For this review, use the dimensioned drawing (mm, ordinates from the lowest corner) and the shaded views. Coordinates: 2 decimals unless noted, no trailing zeros. Loops run counter-clockwise (first coordinate to the right, second up) from the corner with the lowest first, then second, coordinate; pieces in that order, holes last. Notation, with made-up numbers: M 14,62.25 L 32,62.25 A18 ccw 32,87.25 Z; hole C 30.25,79 d2. An arc over 180 degrees is marked long. Write item = value, one per line.
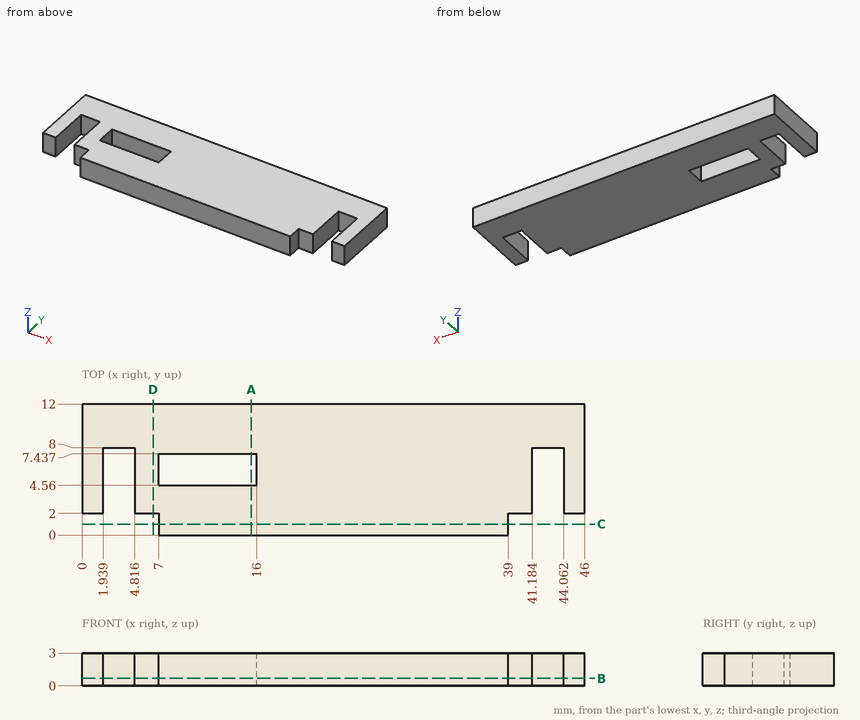
Q1. Add section B-B (z = 0.7). Write out the cut boundary in (x, y) (1 decimal).
Solved:
outline = M 0,2 L 1.9,2 L 1.9,8 L 4.8,8 L 4.8,2 L 7,2 L 7,0 L 39,0 L 39,2 L 41.2,2 L 41.2,8 L 44.1,8 L 44.1,2 L 46,2 L 46,12 L 0,12 Z; hole M 7,4.6 L 16,4.6 L 16,7.4 L 7,7.4 Z
Q2. For line 1 along X through (y, z) = (7, 0.7) (1 decimal); line 2 along X through (y, z) = (2.5, 2.85) (1 decimal); line 3 along Y through (x, z) = (13, 2.25), list the stretches that pass through material, from the lowest coordinate up.
Solved:
line_1 = 0 to 1.9, 4.8 to 7, 16 to 41.2, 44.1 to 46
line_2 = 0 to 1.9, 4.8 to 41.2, 44.1 to 46
line_3 = 0 to 4.56, 7.44 to 12
Q3. Add section D-D (x = 6.5). Write out the cut boundary in (y, z), and give its area (3 significant figures).
Solved:
outline = M 2,0 L 12,0 L 12,3 L 2,3 Z
area = 30.0 mm²
Q4. For pin 1 Ø0.6 at (x, z) = (45.5, 1) entering from -Y; pin 2 Ø1.4 at (x, z) = (3.5, 1) entering from -Y; pin 3 Ø0.6 at (y, z) = (0.5, 2) entering from +X, all flat-tipped, find the tip position at first contact; note any pin that passes through.
Solved:
pin_1 = 2
pin_2 = 8
pin_3 = 39
Q5. Add section A-A (x = 15.5). Write out the cut boundary in (y, z).
Solved:
outline = M 0,0 L 4.56,0 L 4.56,3 L 0,3 Z; M 7.44,0 L 12,0 L 12,3 L 7.44,3 Z
Q6. Add section C-C (y = 1). Write out the cut boundary in (x, z).
Solved:
outline = M 7,0 L 39,0 L 39,3 L 7,3 Z
